Here's the drawing with two shaded views (mm, measured from the low corner). I have some questions. Coordinates: 2 decimals unless noted, no trailing zeros. Order: outer loops, then holes, each group sorted by start corner. A loop starts at its lowest first (then second) coordinate and runs counter-clockwise, first axis right, second up. Notation, with made-up numbers: (-10, 57) -> (44, 57) arc R17 ccw to (44, 90) -> close; hole circle Ø9 at (3.25, 75.25). An arc over 180 degrees is marked (long way). Answer as a JSON object with one key per item and string values. Group by question number.
(1) I need wall thicknesses on line 1 (X direction, y = 1, z = 134) (1 decimal); line 2 (X direction, y = 11.25, z = 90); line 3 (Y direction, x = 40.5, z = 29). Which ranges of each line are inside material? Lowest first, please.
(2) For pin 1 (6 mm diameter, centred on y = 11.5, z = 89, fed in from -X); pin 2 (1.5 mm diameter, centred on x = 84, z = 58, fed in from -Y); pin 3 (3 mm diameter, centred on y = 3.5, z = 85.5, fed in from -X); pin 4 (3 mm diameter, centred on x = 90.5, z = 90.5, fed in from +Y), each with a flat end and sliding along its axis, tell me the tip position at first contact or that it passes through.
(3) I want a section at B-B, the plane x = 27. List the corners of the cut face in (y, z) for me (1 decimal).
(4) I want a section at C-C, the plane z = 67. List the corners of the cut face in (x, y) for me (1 decimal).
(5) I want a section at A-A, the plane x = 59. List the corners of the cut face in (y, z) for me.
(6) I want a section at D-D, the plane x = 103. List the corners of the cut face in (y, z) for me (1 decimal).
(7) If we mould it in two halves opening along Z, with no side actions, what happens to the marked faces 1 and 2? For each: pulls with the +Z half, pulls with the -Z half, needs draft (parallel to the pull), parting line crosses it, or undercut.
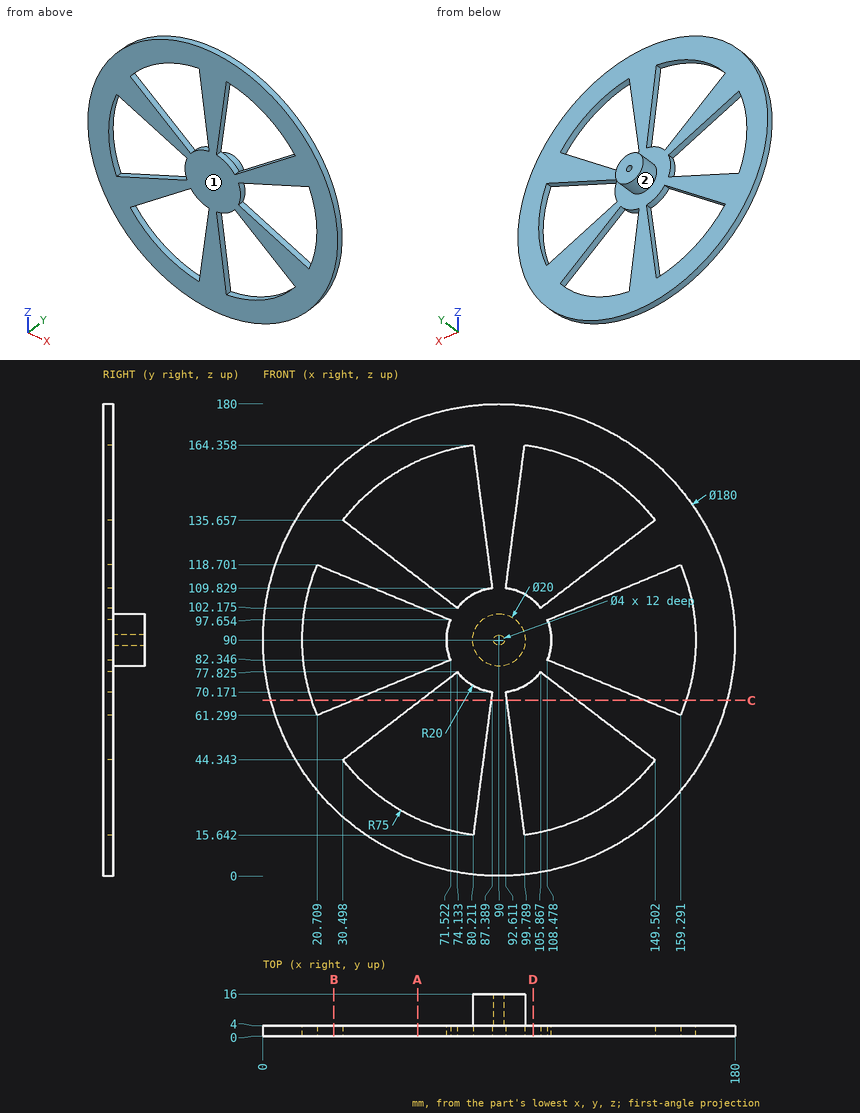
Computed values:
{
 "1": {"line 1": "x = 11.5 to 32.7, 84.2 to 95.8, 147.3 to 168.5", "line 2": "x = 80 to 88, 92 to 100", "line 3": "y = 0 to 4"},
 "2": {"pin 1": "stops at x = 80", "pin 2": "passes through", "pin 3": "stops at x = 0.05", "pin 4": "stops at y = 16"},
 "3": {"outline": "(0, 25.7) -> (4, 25.7) -> (4, 63.9) -> (0, 63.9) -> close; (0, 116.1) -> (4, 116.1) -> (4, 154.3) -> (0, 154.3) -> close"},
 "4": {"outline": "(3, 0) -> (18.6, 0) -> (18.6, 4) -> (3, 4) -> close; (34.5, 0) -> (60, 0) -> (60, 4) -> (34.5, 4) -> close; (87, 0) -> (93, 0) -> (93, 4) -> (87, 4) -> close; (120, 0) -> (145.5, 0) -> (145.5, 4) -> (120, 4) -> close; (161.4, 0) -> (177, 0) -> (177, 4) -> (161.4, 4) -> close"},
 "5": {"outline": "(0, 5.51) -> (4, 5.51) -> (4, 21.71) -> (0, 21.71) -> close; (0, 66.21) -> (4, 66.21) -> (4, 77.16) -> (0, 77.16) -> close; (0, 102.84) -> (4, 102.84) -> (4, 113.79) -> (0, 113.79) -> close; (0, 158.29) -> (4, 158.29) -> (4, 174.49) -> (0, 174.49) -> close"},
 "6": {"outline": "(0, 0.9) -> (4, 0.9) -> (4, 16.1) -> (0, 16.1) -> close; (0, 74.8) -> (4, 74.8) -> (4, 105.2) -> (0, 105.2) -> close; (0, 163.9) -> (4, 163.9) -> (4, 179.1) -> (0, 179.1) -> close"},
 "7": {"face 1": "needs draft", "face 2": "parting line crosses it"}
}
